Verification items for this drawing (mm, ordinates from the low corner). Give positions to 0.01 mm unless a question says otherwise; leave off trailing zeros. Loops run counter-clockwise (first coordinate to the right, second up) from the corner with the lowest first, then second, coordinate; pieces in that order, holes last. Notation, with made-up numbers: (51.5, -3) -> (60.5, -3) arc R12 ccw to (60.5, 5) -> close; hole circle Ø9 at (81.5, -11.75). An arc over 180 degrees is marked (long way). Write each question's results on one line, items separated by ' | '. Start each with the question number.
1) Depth check by flat-ended pin: pin 1 (1.5 mm diameter, centred on x = 13.97, y = 13.97, fed in from -Z). Enter the tip coordinate at first touch or a pass-through.
2) Sectioned sample at C-C on x = 1.5. Record the cut outline in (y, z), then the cut area to 3 significant figures.
3) Draft check along Y on the marked faces 1, 2 and 3. Enter one of: pulls with the +Y half, pulls with the -Y half, needs draft (parallel to the pull), parting line crosses it, or undercut.
4) Sectioned sample at B-B on y = 14.5. Record the cut outline in (x, z).
5) Sectioned sample at A-A on z = 1.1. Record the cut outline in (x, y) (3 decimals), then the cut area to 3 significant figures.
6) Scan lines: line 1 (Y direction, x = 13.97, z = 1.05); line 2 (Y direction, x = 3, z = 0.4); line 3 (Y direction, x = 13.25, z = 1.45). Record each from-to range of solid material in increasing order. Write a range as from..to.
7) Sectioned sample at D-D on x = 14.5. Record the cut outline in (y, z).
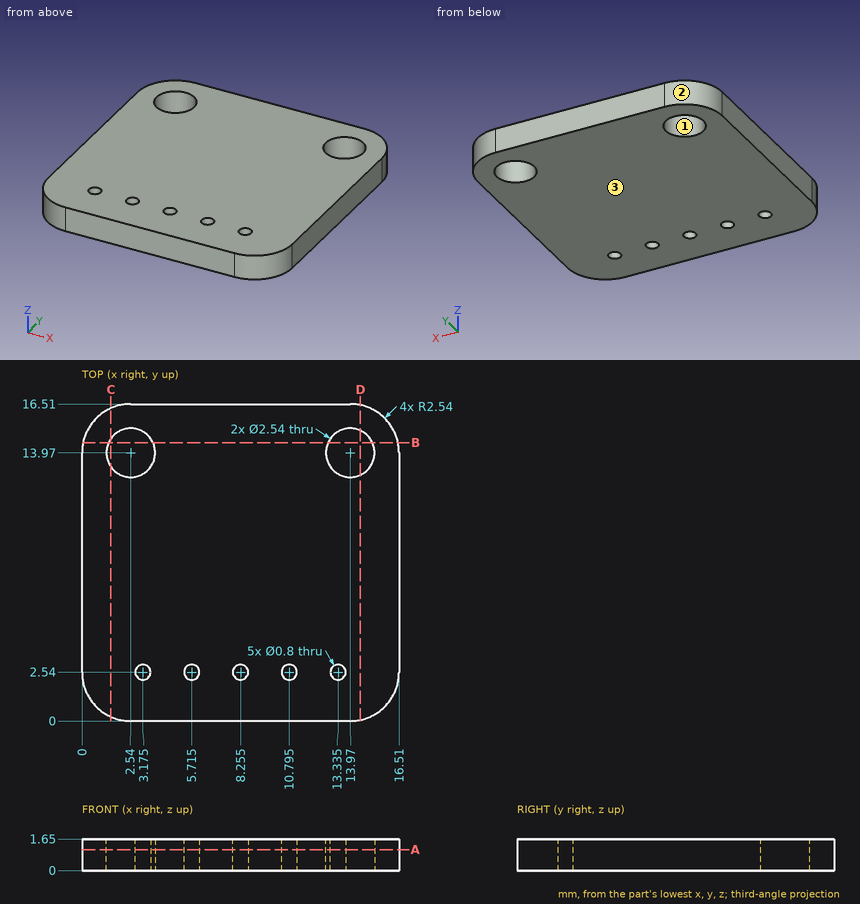
Result:
1) pin 1: through
2) outline: (0.22, 0) -> (13.24, 0) -> (13.24, 1.65) -> (0.22, 1.65) -> close; (14.7, 0) -> (16.29, 0) -> (16.29, 1.65) -> (14.7, 1.65) -> close | area: 24.1 mm^2
3) face 1: undercut | face 2: pulls with the +Y half | face 3: needs draft
4) outline: (0.06, 0) -> (1.39, 0) -> (1.39, 1.65) -> (0.06, 1.65) -> close; (3.69, 0) -> (12.82, 0) -> (12.82, 1.65) -> (3.69, 1.65) -> close; (15.12, 0) -> (16.45, 0) -> (16.45, 1.65) -> (15.12, 1.65) -> close
5) outline: (0, 2.54) arc R2.54 ccw to (2.54, 0) -> (13.97, 0) arc R2.54 ccw to (16.51, 2.54) -> (16.51, 13.97) arc R2.54 ccw to (13.97, 16.51) -> (2.54, 16.51) arc R2.54 ccw to (0, 13.97) -> close; hole circle Ø2.54 at (2.54, 13.97); hole circle Ø0.8 at (3.175, 2.54); hole circle Ø0.8 at (5.715, 2.54); hole circle Ø0.8 at (8.255, 2.54); hole circle Ø0.8 at (10.795, 2.54); hole circle Ø2.54 at (13.97, 13.97); hole circle Ø0.8 at (13.335, 2.54) | area: 254 mm^2
6) line 1: 0..12.7, 15.24..16.51 | line 2: 0..2.18, 2.9..12.79, 15.15..16.51 | line 3: 0..2.15, 2.93..12.92, 15.02..16.51
7) outline: (0.06, 0) -> (12.82, 0) -> (12.82, 1.65) -> (0.06, 1.65) -> close; (15.12, 0) -> (16.45, 0) -> (16.45, 1.65) -> (15.12, 1.65) -> close
